Read the model definition and answer for the solid it produces. Units are mm, in the model's axes. A direction names the side the tool comes from. Give positions to 0.01 mm unless a question says otherwise; leave off trailing zeros. Order: outer loops, then holes, each group sorted by start corner. A loop starts at its lowest first (then second) coordinate and runs counter-clockwise, first axis right, second up.
```python
from build123d import *

# Parameters (mm, degrees)
BOSS_EXTRUDE1_DEPTH = 101.6


with BuildPart() as part:
    # Sketch1 → Boss-Extrude1 (new body)
    with BuildSketch(Plane(origin=(0, 0, 0), x_dir=(1, 0, 0), z_dir=(0, 1, 0))):
        with BuildLine():
            Line((-61.89337695, 68.904893678), (-61.89337695, 82.620893678))
            ThreePointArc((-61.89337695, 82.620893678), (-57.499978668, 93.227495396), (-46.89337695, 97.620893678))
            Line((-46.89337695, 97.620893678), (44.10662305, 97.620893678))
            ThreePointArc((44.10662305, 97.620893678), (54.713224768, 93.227495396), (59.10662305, 82.620893678))
            Line((59.10662305, 82.620893678), (59.10662305, 71.13235))
            ThreePointArc((59.10662305, 71.13235), (68.479206052, 48.504933002), (91.10662305, 39.13235))
            Line((91.10662305, 39.13235), (94.60662305, 39.13235))
            ThreePointArc((94.60662305, 39.13235), (105.213224768, 34.738951718), (109.60662305, 24.13235))
            Line((109.60662305, 24.13235), (109.60662305, -24.13235))
            ThreePointArc((109.60662305, -24.13235), (105.213224768, -34.738951718), (94.60662305, -39.13235))
            Line((94.60662305, -39.13235), (91.10662305, -39.13235))
            ThreePointArc((91.10662305, -39.13235), (68.479206052, -48.504933002), (59.10662305, -71.13235))
            Line((59.10662305, -71.13235), (59.10662305, -82.620893678))
            ThreePointArc((59.10662305, -82.620893678), (54.713224768, -93.227495396), (44.10662305, -97.620893678))
            Line((44.10662305, -97.620893678), (-46.89337695, -97.620893678))
            ThreePointArc((-46.89337695, -97.620893678), (-57.499978668, -93.227495396), (-61.89337695, -82.620893678))
            Line((-61.89337695, -82.620893678), (-61.89337695, -68.904893678))
            ThreePointArc((-61.89337695, -68.904893678), (-57.006333295, -61.056893678), (-47.807345705, -61.98043415))
            ThreePointArc((-47.807345705, -61.98043415), (1.776e-06, -78.2759), (47.807348518, -61.98043198))
            ThreePointArc((47.807348518, -61.98043198), (49.925699103, -59.785267241), (51.321425315, -57.072684381))
            ThreePointArc((51.321425315, -57.072684381), (58.006985995, -44.607187443), (68.337697819, -34.944800122))
            ThreePointArc((68.337697819, -34.944800122), (70.600912289, -32.899312969), (72.178496552, -30.288300651))
            ThreePointArc((72.178496552, -30.288300651), (78.2759, -7.06e-07), (72.178497098, 30.288299349))
            ThreePointArc((72.178497098, 30.288299349), (70.600912642, 32.899311988), (68.337697819, 34.94479931))
            ThreePointArc((68.337697819, 34.94479931), (58.006984392, 44.607187472), (51.321422969, 57.072685993))
            ThreePointArc((51.321422969, 57.072685993), (49.92569661, 59.785269199), (47.807345705, 61.98043415))
            ThreePointArc((47.807345705, 61.98043415), (0, 78.2759), (-47.807345705, 61.98043415))
            ThreePointArc((-47.807345705, 61.98043415), (-57.006333295, 61.056893678), (-61.89337695, 68.904893678))
        make_face()
    extrude(amount=BOSS_EXTRUDE1_DEPTH)


solid = part.part
```
1) A tool of negligible diameter and unlimited length cuts with its end or side. For faces 1 (the face through (49.9, 50.09, 59.82)), 2 (the face through (78.275, 50.089, 0.435)), 3 (the face through (59.107, 50, 77)), from which of +Z, -Z, +X, -X, +Y, -Y can it reach the whole face along a straight path? Write none if from no direction.
Final values:
face 1: +Y, -Y
face 2: -X, +Y, -Y
face 3: +Z, +X, +Y, -Y
2) The part is cut by section B-B on y = 95. Determine the outline of the cut face in (x, z) (1 decimal), and give its area (3 significant figures).
Final values:
outline: (-61.9, -82.6) arc R15 ccw to (-46.9, -97.6) - (44.1, -97.6) arc R15 ccw to (59.1, -82.6) - (59.1, -71.1) arc R32 cw to (91.1, -39.1) - (94.6, -39.1) arc R15 ccw to (109.6, -24.1) - (109.6, 24.1) arc R15 ccw to (94.6, 39.1) - (91.1, 39.1) arc R32 cw to (59.1, 71.1) - (59.1, 82.6) arc R15 ccw to (44.1, 97.6) - (-46.9, 97.6) arc R15 ccw to (-61.9, 82.6) - (-61.9, 68.9) arc R8.7 ccw to (-47.8, 62) arc R78.3 cw to (47.8, 62) arc R10.5 cw to (51.3, 57.1) arc R43.5 ccw to (68.3, 34.9) arc R10.5 cw to (72.2, 30.3) arc R78.3 cw to (72.2, -30.3) arc R10.5 cw to (68.3, -34.9) arc R43.5 ccw to (51.3, -57.1) arc R10.5 cw to (47.8, -62) arc R78.3 cw to (-47.8, -62) arc R8.7 ccw to (-61.9, -68.9) - close
area: 9,610 mm2
3) Given pin 1 (3 mm diameter, centred on y = 36.5, z = 47, fed in from -X); pin 2 (9 mm diameter, centred on y = 49, z = -78, fed in from +X); pin 3 (6 mm diameter, centred on y = 60, z = -22.5, fed in from -X), each flat-ended and moving along its own axis, determine where each tip first touches the part or whether it passes through.
Final values:
pin 1: stops at x = 55.34
pin 2: stops at x = 59.11
pin 3: stops at x = 74.01
4) The part is cut by section D-D on z = -12. Determine the outline of the cut face in (x, y), and give its area (3 significant figures).
Final values:
outline: (77.35, 0) - (109.61, 0) - (109.61, 101.6) - (77.35, 101.6) - close
area: 3,280 mm2
5) The part is cut by section C-C on x = 63. Determine the outline of the cut face in (y, z).
Final values:
outline: (0, -55.83) - (101.6, -55.83) - (101.6, -39.15) - (0, -39.15) - close; (0, 39.15) - (101.6, 39.15) - (101.6, 55.83) - (0, 55.83) - close
6) Consider L1, parallel to Z at x = -24, y = 62; L2, parallel to Z at x = 62, y = 61; L3, parallel to X at y = 79, z = 81. Determine where each line is inside the solid, lowest interval first.
Final values:
L1: z = -97.62 to -74.51, 74.51 to 97.62
L2: z = -57.84 to -40.1, 40.1 to 57.84
L3: x = -61.89 to 59.11
7) For a pull along X with two mould halves and no side action, classify faces 4 (the face through (-56.883, 50.089, -60.998)), 5 (the face through (57.886, 50.089, 44.765)), 6 (the face through (68.232, 50.089, -48.755)) as released by +X, released by -X, zero draft, split by the parting line, or undercut.
Final values:
face 4: undercut
face 5: released by -X
face 6: released by +X
8) The part is cut by section A-A on x = -36. Determine the outline of the cut face in (y, z), and give its area (3 significant figures).
Final values:
outline: (0, -97.62) - (101.6, -97.62) - (101.6, -69.51) - (0, -69.51) - close; (0, 69.51) - (101.6, 69.51) - (101.6, 97.62) - (0, 97.62) - close
area: 5,710 mm2
